```python
from build123d import *

# Parameters (mm, degrees)
SKETCH_1_W             = 130
SKETCH_1_H             = 130
EXTRUDE_1_DEPTH        = 40.6
SKETCH_2_W             = 130
SKETCH_2_H             = 40.5
CUT_EXTRUDE_1_DEPTH    = 24
SKETCH_7_W             = 16
SKETCH_7_H             = 30
CUT_EXTRUDE_5_DEPTH    = 20
CUT_EXTRUDE_8_DEPTH    = 10
HOLE_WIZARD_M2_1_D     = 1.6
HOLE_WIZARD_M2_1_DEPTH = 8
HOLE_WIZARD_M2_1_TIP   = 0.480688495
SKETCH_15_W            = 100
SKETCH_15_H            = 100
CUT_EXTRUDE_9_DEPTH    = 5
FILLET_1_R             = 10
HOLE_WIZARD_M2_3_D     = 1.6
HOLE_WIZARD_M2_3_DEPTH = 8
HOLE_WIZARD_M2_3_TIP   = 0.480688495
SKETCH_24_W            = 68
SKETCH_24_H            = 30.5
CUT_EXTRUDE_10_DEPTH   = 20
SKETCH_25_W            = 4
SKETCH_25_H            = 16
CUT_EXTRUDE_11_DEPTH   = 25
SKETCH_26_W            = 31
SKETCH_26_H            = 20
CUT_EXTRUDE_12_DEPTH   = 20
SKETCH_27_R            = 2.5
EXTRUDE_2_DEPTH        = 2
SKETCH_28_W            = 70
SKETCH_28_H            = 35
CUT_EXTRUDE_13_DEPTH   = 15
SKETCH_29_W            = 110
SKETCH_29_H            = 110
CUT_EXTRUDE_14_DEPTH   = 10
SKETCH_30_R            = 2.5
EXTRUDE_4_DEPTH        = 2
HOLE_WIZARD_M2_4_D     = 1.6
HOLE_WIZARD_M2_4_DEPTH = 8
HOLE_WIZARD_M2_4_TIP   = 0.480688495
HOLE_WIZARD_M3_1_D     = 2.5
HOLE_WIZARD_M3_1_DEPTH = 8
HOLE_WIZARD_M3_1_TIP   = 0.751075774
HOLE_WIZARD_M2_7_D     = 1.6
HOLE_WIZARD_M2_7_DEPTH = 8
HOLE_WIZARD_M2_7_TIP   = 0.480688495


with BuildPart() as part:
    # 草图1 → 凸台-拉伸1 (new body)
    with BuildSketch(Plane(origin=(0, 0, 0), x_dir=(1, 0, 0), z_dir=(0, 1, 0))):
        Rectangle(SKETCH_1_W, SKETCH_1_H)
    extrude(amount=EXTRUDE_1_DEPTH)

    # 草图2 → 切除-拉伸1 (cut)
    with BuildSketch(Plane(origin=(0, 40.6, 0), x_dir=(1, 0, 0), z_dir=(0, 1, 0))):
        with Locations((0, 36.75)):
            Rectangle(SKETCH_2_W, SKETCH_2_H)
    extrude(amount=-CUT_EXTRUDE_1_DEPTH, mode=Mode.SUBTRACT)

    # 草图7 → 切除-拉伸5 (cut)
    with BuildSketch(Plane.XZ):
        with Locations((57, 0)):
            Rectangle(SKETCH_7_W, SKETCH_7_H)
        with Locations((-57, 0)):
            Rectangle(SKETCH_7_W, SKETCH_7_H)
    extrude(amount=-CUT_EXTRUDE_5_DEPTH, mode=Mode.SUBTRACT)

    # 草图10 → 切除-拉伸8 (cut)
    with BuildSketch(Plane.XZ):
        with BuildLine():
            Line((-41, -50), (41, -50))
            ThreePointArc((41, -50), (44.535533906, -48.535533906), (46, -45))
            Line((46, -45), (46, 19))
            ThreePointArc((46, 19), (44.535533906, 22.535533906), (41, 24))
            Line((41, 24), (-41, 24))
            ThreePointArc((-41, 24), (-44.535533906, 22.535533906), (-46, 19))
            Line((-46, 19), (-46, -45))
            ThreePointArc((-46, -45), (-44.535533906, -48.535533906), (-41, -50))
        make_face()
    extrude(amount=-CUT_EXTRUDE_8_DEPTH, mode=Mode.SUBTRACT)

    # M2 螺纹孔的螺纹孔钻头1
    with Locations(Plane(origin=(0, 0, 0), x_dir=(-1, 0, 0), z_dir=(0, -1, 0))):
        with Locations((60, -60), (-60, -60), (60, 60), (-60, 60)):
            Hole(HOLE_WIZARD_M2_1_D / 2, depth=HOLE_WIZARD_M2_1_DEPTH)
            with Locations((0, 0, -(HOLE_WIZARD_M2_1_DEPTH + HOLE_WIZARD_M2_1_TIP / 2))):  # 118° drill point
                Cone(0, HOLE_WIZARD_M2_1_D / 2, HOLE_WIZARD_M2_1_TIP, mode=Mode.SUBTRACT)

    # 草图15 → 切除-拉伸9 (cut)
    with BuildSketch(Plane.XZ):
        Rectangle(SKETCH_15_W, SKETCH_15_H)
    extrude(amount=-CUT_EXTRUDE_9_DEPTH, mode=Mode.SUBTRACT)

    # 圆角1
    fillet_1_edges = [part.edges().sort_by_distance(p)[0] for p in [
        (65, 20.3, 65),
        (-65, 20.3, 65),
        (-65, 20.3, -65),
        (65, 20.3, -65),
    ]]
    fillet(fillet_1_edges, radius=FILLET_1_R)

    # M2 螺纹孔的螺纹孔钻头3
    with Locations(Plane(origin=(0, 40.6, 0), x_dir=(1, 0, 0), z_dir=(0, 1, 0))):
        with Locations((-60, 60), (60, 60), (60, -60), (-60, -60)):
            Hole(HOLE_WIZARD_M2_3_D / 2, depth=HOLE_WIZARD_M2_3_DEPTH)
            with Locations((0, 0, -(HOLE_WIZARD_M2_3_DEPTH + HOLE_WIZARD_M2_3_TIP / 2))):  # 118° drill point
                Cone(0, HOLE_WIZARD_M2_3_D / 2, HOLE_WIZARD_M2_3_TIP, mode=Mode.SUBTRACT)

    # 草图24 → 切除-拉伸10 (cut)
    with BuildSketch(Plane(origin=(0, 40.6, 0), x_dir=(1, 0, 0), z_dir=(0, 1, 0))):
        with Locations((0, -49.75)):
            Rectangle(SKETCH_24_W, SKETCH_24_H)
    extrude(amount=-CUT_EXTRUDE_10_DEPTH, mode=Mode.SUBTRACT)

    # 草图25 → 切除-拉伸11 (cut)
    with BuildSketch(Plane(origin=(0, 40.6, 0), x_dir=(1, 0, 0), z_dir=(0, 1, 0))):
        with Locations((-36, -48.559593505)):
            Rectangle(SKETCH_25_W, SKETCH_25_H)
    extrude(amount=-CUT_EXTRUDE_11_DEPTH, mode=Mode.SUBTRACT)

    # 草图26 → 切除-拉伸12 (cut)
    with BuildSketch(Plane(origin=(0, 40.6, 0), x_dir=(1, 0, 0), z_dir=(0, 1, 0))):
        with Locations((49.5, -44.5)):
            Rectangle(SKETCH_26_W, SKETCH_26_H)
    extrude(amount=-CUT_EXTRUDE_12_DEPTH, mode=Mode.SUBTRACT)

    # 草图27 → 凸台-拉伸2 (add)
    with BuildSketch(Plane(origin=(0, 20.6, 0), x_dir=(1, 0, 0), z_dir=(0, 1, 0))):
        with Locations(Location((30.5, -61.75, 0), (0, 0, 270))):
            Circle(SKETCH_27_R)
        with Locations(Location((-22.51, -61.75, 0), (0, 0, 270))):
            Circle(SKETCH_27_R)
        with Locations(Location((-22.51, -37.74, 0), (0, 0, 270))):
            Circle(SKETCH_27_R)
    extrude(amount=EXTRUDE_2_DEPTH)

    # 草图28 → 切除-拉伸13 (cut)
    with BuildSketch(Plane(origin=(0, 40.6, 0), x_dir=(1, 0, 0), z_dir=(0, 1, 0))):
        with Locations((0.006580057, -4.600945461)):
            Rectangle(SKETCH_28_W, SKETCH_28_H)
    extrude(amount=-CUT_EXTRUDE_13_DEPTH, mode=Mode.SUBTRACT)

    # 草图29 → 切除-拉伸14 (cut)
    with BuildSketch(Plane(origin=(0, 40.6, 0), x_dir=(1, 0, 0), z_dir=(0, 1, 0))):
        Rectangle(SKETCH_29_W, SKETCH_29_H)
    extrude(amount=-CUT_EXTRUDE_14_DEPTH, mode=Mode.SUBTRACT)

    # 草图30 → 凸台-拉伸4 (add)
    with BuildSketch(Plane.XZ.offset(-10)):
        with Locations(Location((40, 18, 0), (0, 0, 90))):
            Circle(SKETCH_30_R)
        with Locations(Location((40, -44, 0), (0, 0, 90))):
            Circle(SKETCH_30_R)
        with Locations(Location((-40, -44, 0), (0, 0, 90))):
            Circle(SKETCH_30_R)
        with Locations(Location((-40, 18, 0), (0, 0, 90))):
            Circle(SKETCH_30_R)
    extrude(amount=EXTRUDE_4_DEPTH)

    # M2 螺纹孔的螺纹孔钻头4
    with Locations(Plane(origin=(0, 0, -65), x_dir=(-1, 0, 0), z_dir=(0, 0, -1))):
        with Locations((-29.333554251, 23.053823954), (-14.333768955, 23.134080314), (21.033223503, 20.063926498), (35, 19.1)):
            Hole(HOLE_WIZARD_M2_4_D / 2, depth=HOLE_WIZARD_M2_4_DEPTH)
            with Locations((0, 0, -(HOLE_WIZARD_M2_4_DEPTH + HOLE_WIZARD_M2_4_TIP / 2))):  # 118° drill point
                Cone(0, HOLE_WIZARD_M2_4_D / 2, HOLE_WIZARD_M2_4_TIP, mode=Mode.SUBTRACT)

    # M3 螺纹孔的螺纹孔钻头1
    with Locations(Plane(origin=(0, 8, 0), x_dir=(-1, 0, 0), z_dir=(0, -1, 0))):
        with Locations((40, -18), (-40, -18), (40, 44), (-40, 44)):
            Hole(HOLE_WIZARD_M3_1_D / 2, depth=HOLE_WIZARD_M3_1_DEPTH)
            with Locations((0, 0, -(HOLE_WIZARD_M3_1_DEPTH + HOLE_WIZARD_M3_1_TIP / 2))):  # 118° drill point
                Cone(0, HOLE_WIZARD_M3_1_D / 2, HOLE_WIZARD_M3_1_TIP, mode=Mode.SUBTRACT)

    # M2 螺纹孔的螺纹孔钻头7
    with Locations(Plane(origin=(0, 22.6, 0), x_dir=(1, 0, 0), z_dir=(0, 1, 0))):
        with Locations((-22.51, -37.74), (-22.51, -61.75), (30.5, -61.75)):
            Hole(HOLE_WIZARD_M2_7_D / 2, depth=HOLE_WIZARD_M2_7_DEPTH)
            with Locations((0, 0, -(HOLE_WIZARD_M2_7_DEPTH + HOLE_WIZARD_M2_7_TIP / 2))):  # 118° drill point
                Cone(0, HOLE_WIZARD_M2_7_D / 2, HOLE_WIZARD_M2_7_TIP, mode=Mode.SUBTRACT)


solid = part.part
```
Work out the finished part from the listing and answer in its coordinate system (mm). A direction names the side the tool comes from. Round coordinates to 2 decimals unless told otherwise and drop trailing zeros. Order: outer loops, then holes, each group sorted by start corner. A loop starts at its lowest first (then second) coordinate and runs counter-clockwise, first axis right, second up.
Q1. A cutting plane is placed at A-A, the plane z = -3. Determine the outline of the cut face in (x, y), then the cut area to 3 significant figures.
Solution:
outline: (-65, 20) - (-49, 20) - (-49, 5) - (-46, 5) - (-46, 10) - (46, 10) - (46, 5) - (49, 5) - (49, 20) - (65, 20) - (65, 40.6) - (55, 40.6) - (55, 30.6) - (35.01, 30.6) - (35.01, 25.6) - (-34.99, 25.6) - (-34.99, 30.6) - (-55, 30.6) - (-55, 40.6) - (-65, 40.6) - close
area: 2,240 mm2
Q2. Find the intervals of material crossed by line 1 along Z through (x, y) = (57, 21.5); line 2 along Z through (x, y) = (-36, 18); line 3 along Z through (x, y) = (18, 3.5), in increasing order.
Solution:
line 1: z = -64.8 to -57, -16.5 to 34.5, 54.5 to 64.8
line 2: z = -65 to -57, -16.5 to 40.56, 56.56 to 65
line 3: z = -65 to -50, 50 to 65
Q3. A cutting plane is placed at B-B, the plane x = 11. Determine the outline of the cut face in (y, z).
Solution:
outline: (0, -65) - (40.6, -65) - (40.6, -57) - (16.6, -57) - (16.6, -16.5) - (30.6, -16.5) - (30.6, -12.9) - (25.6, -12.9) - (25.6, 22.1) - (30.6, 22.1) - (30.6, 34.5) - (20.6, 34.5) - (20.6, 65) - (0, 65) - (0, 50) - (5, 50) - (5, 24) - (10, 24) - (10, -50) - (0, -50) - close
Q4. Given pin 1 Ø4 at (x, z) = (-39.5, -44.5) entering from -Y; pin 2 Ø3 at (x, z) = (-40, 18) entering from +Y; pin 3 Ø10 at (x, y) = (-12.5, 32.5) entering from +Z; pin 4 Ø1.8 at (x, z) = (60, -60) entering from -Y, each flat-ended and moving along its own axis, determine where each tip first touches the part or whether it passes through.
Solution:
pin 1: stops at y = 8
pin 2: stops at y = 30.6
pin 3: stops at z = 34.5
pin 4: stops at y = 0
Q5. The mould has two halves that part along Z. Classify faces 1 (the flat face through (-24, 22.6, 62)), 2 (the flat face through (-1, 29, -57)), 3 (the cylindrical face through (62.15, 20.58, -61.99)): pulls with the +Z half, pulls with the -Z half, needs draft (parallel to the pull), parting line crosses it, or undercut.
Solution:
face 1: needs draft
face 2: undercut
face 3: pulls with the -Z half
Q6. A tool of negligible diameter and unlimited length cuts with its end or side. For faces 4 (the cylindrical face through (-44, 7, 23)), 5 (the cylindrical face through (-62.15, 20.58, 61.99)), 6 (the flat face through (-34, 26, 38)), 7 (the flat face through (-38, 23, 49)), from which of +Z, -Z, +X, -X, +Y, -Y can it reach the whole face along a straight path? Write none if from no direction.
Solution:
face 4: -Y
face 5: +Z, -X, +Y, -Y
face 6: +Z, +Y
face 7: +Y
